```python
from build123d import *

# Parameters (mm, degrees)
F0_W     = 80
F0_H     = 20
F0_W_2   = 62.5
F0_H_2   = 0.825
F1_DEPTH = 6
F2_R     = 9.99999


# Not quite as in the source:
# - a fillet or chamfer is up to 0.001 mm smaller than in the source, because OpenCascade refuses the exact size


with BuildPart() as f1:
    # F0 (on Top) → F1 (new body)
    with BuildSketch(Plane.XY):
        Rectangle(F0_W, F0_H)
        Rectangle(F0_W_2, F0_H_2, mode=Mode.SUBTRACT)
    extrude(amount=F1_DEPTH)

    # F2 (radius 10 in the source; OpenCascade refuses exactly that, so slightly less here)
    f2_edges = [f1.edges().sort_by_distance(p)[0] for p in [
        (-40, 10, 3),
        (-40, -10, 3),
        (40, 10, 3),
        (40, -10, 3),
    ]]
    fillet(f2_edges, radius=F2_R)


solid = f1.part
```
Input: part model. Units: mm. Frame: model coordinates. Round coordinates to 2 decimals unless told otherwise and drop trailing zeros. Loops run counter-clockwise (first coordinate to the right, second up) from the corner with the lowest first, then second, coordinate; pieces in that order, holes last.
1) Section query D-D on y = 3.5. Return the cut outline in (x, z).
Ans:
outline: (-39.37, 0) - (39.37, 0) - (39.37, 6) - (-39.37, 6) - close
2) Section query C-C on y = -6.75. Return the cut outline in (x, z), plus the area to 3 significant figures.
Ans:
outline: (-37.38, 0) - (37.38, 0) - (37.38, 6) - (-37.38, 6) - close
area: 449 mm2
3) Pull-direction query (Y, two-part tool) for faces 1 (the flat face through (0, -0.412, 3)), 2 (the cylindrical face through (36.99, -7.15, 3.04)), 3 (the flat face through (0, 0.412, 3)), 4 (the flat face through (-1, 2, 0)); classes: released by +Y, released by -Y, zero draft, split by the parting line, or undercut.
Ans:
face 1: undercut
face 2: released by -Y
face 3: undercut
face 4: zero draft
4) Pin query (flat end, axial travel): pin 1 (1.5 mm diameter, centred on y = 4, z = 5.5, fed in from +X). Return the tip coordinate at first contact, or that it passes through.
Ans:
pin 1: stops at x = 39.46
5) Material intervals for line 1 (Y direction, x = 14, z = 5.15); line 2 (X direction, y = -2.75, z = 3.1); line 3 (X direction, y = -6.75, z = 4), sorted ascending.
Ans:
line 1: y = -10 to -0.41, 0.41 to 10
line 2: x = -39.61 to 39.61
line 3: x = -37.38 to 37.38
6) Section query A-A on x = -20.5. Return the cut outline in (y, z), plus the area to 3 significant figures.
Ans:
outline: (-10, 0) - (-0.41, 0) - (-0.41, 6) - (-10, 6) - close; (0.41, 0) - (10, 0) - (10, 6) - (0.41, 6) - close
area: 115 mm2
